Read the model definition and answer for the solid it produces. Units are mm, in the model's axes. Face numbers are marked on the shaded views. Round coordinates to 2 decimals unless told otherwise and drop trailing zeros. Order: outer loops, then holes, each group sorted by start corner. A loop starts at its lowest first (then second) coordinate and runs counter-clockwise, first axis right, second up. Notation, with made-up numbers: (83, 48) -> (109, 48) arc R24 ccw to (109, 65) -> close; hole circle Ø10 at (76, -25.75). An arc over 180 degrees is marked (long way). Use a Markdown table: item, result. Add a question column.
1. Section B-B, the plane y = 21 is taken. Give the vertices of the cut face in (x, z), then the cut area to 3 significant figures.
2. Given pin 1 (4 mm diameter, centred on x = 4.25, y = 4.25, fed in from -Z), flat-ended and moving along its own axis, determine where the tip first touches the part or whether it passes through.
3. Consider L1, parallel to Y at x = 75, z = 8; L2, parallel to X at y = 6, z = 5; L3, parallel to X at y = 49, z = 6. Determine where each line is inside the solid, lowest interval first. Write a range as [from, to].
4. Section D-D, the plane y = 75.75 is taken. Give the vertices of the cut face in (x, z).
5. The mould has two halves that part along X. Classify the marked faces 1, 2, 3 and 4: +X half, -X half, draft (parallel to the pull), parting line (faces both ways), or undercut.
6. Section C-C, the plane z = 2.5 is taken. Give the vertices of the cut face in (x, y).
```python
from build123d import *

# Parameters (mm, degrees)
SKETCH1_W           = 80
SKETCH1_H           = 80
SKETCH1_R           = 38.6
SKETCH1_R_2         = 2.15
BOSS_EXTRUDE1_DEPTH = 25


with BuildPart() as part:
    # Sketch1 → Boss-Extrude1 (new body)
    with BuildSketch(Plane.XY):
        with Locations((40, 40)):
            Rectangle(SKETCH1_W, SKETCH1_H)
        with Locations((40, 40)):
            Circle(SKETCH1_R, mode=Mode.SUBTRACT)
        with Locations((4.25, 75.75)):
            Circle(SKETCH1_R_2, mode=Mode.SUBTRACT)
        with Locations(Location((75.75, 75.75, 0), (0, 0, 180))):
            Circle(SKETCH1_R_2, mode=Mode.SUBTRACT)
        with Locations(Location((4.25, 4.25, 0), (0, 0, 180))):
            Circle(SKETCH1_R_2, mode=Mode.SUBTRACT)
        with Locations((75.75, 4.25)):
            Circle(SKETCH1_R_2, mode=Mode.SUBTRACT)
    extrude(amount=BOSS_EXTRUDE1_DEPTH)


solid = part.part
```
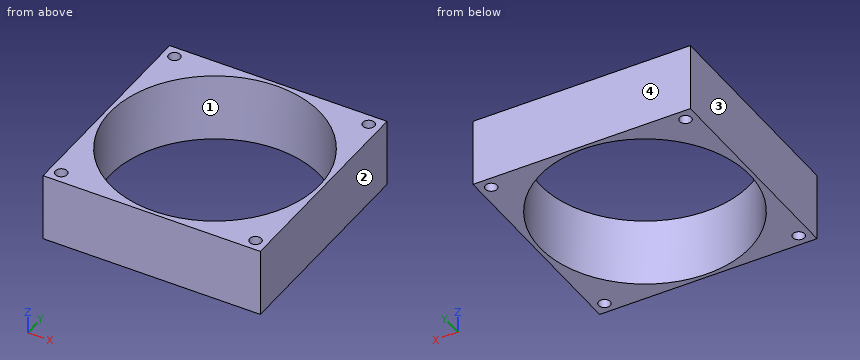
Verdict:
| question | item | result |
|---|---|---|
| 1 | outline | (0, 0) -> (6.4, 0) -> (6.4, 25) -> (0, 25) -> close; (73.6, 0) -> (80, 0) -> (80, 25) -> (73.6, 25) -> close |
| 1 | area | 320 mm2 |
| 2 | pin 1 | passes through |
| 3 | L1 | y = [0, 2.24], [6.26, 23.72], [56.28, 73.74], [77.76, 80] |
| 3 | L2 | x = [0, 3], [5.5, 21.73], [58.27, 74.5], [77, 80] |
| 3 | L3 | x = [0, 2.46], [77.54, 80] |
| 4 | outline | (0, 0) -> (2.1, 0) -> (2.1, 25) -> (0, 25) -> close; (6.4, 0) -> (25.44, 0) -> (25.44, 25) -> (6.4, 25) -> close; (54.56, 0) -> (73.6, 0) -> (73.6, 25) -> (54.56, 25) -> close; (77.9, 0) -> (80, 0) -> (80, 25) -> (77.9, 25) -> close |
| 5 | face 1 | undercut |
| 5 | face 2 | +X half |
| 5 | face 3 | -X half |
| 5 | face 4 | draft |
| 6 | outline | (0, 0) -> (80, 0) -> (80, 80) -> (0, 80) -> close; hole circle Ø77.2 at (40, 40); hole circle Ø4.3 at (4.25, 4.25); hole circle Ø4.3 at (4.25, 75.75); hole circle Ø4.3 at (75.75, 4.25); hole circle Ø4.3 at (75.75, 75.75) |
